```python
from build123d import *

# Parameters (mm, degrees)
SKETCH1_R             = 19.05
BOSS_EXTRUDE1_DEPTH   = 4.7625
SKETCH2_R             = 11.1125
BOSS_EXTRUDE2_DEPTH   = 1.5875
FILLET1_R             = 1.5875
CUT_EXTRUDE1_DEPTH    = 28.679008291
FILLET2_R             = 1.5875
F_4_40_TAPPED_HOLE1_D = 2.2606
CIRPATTERN1_COUNT     = 6
CHAMFER1_SIZE         = 0.762


with BuildPart() as part:
    # Sketch1 → Boss-Extrude1 (new body)
    with BuildSketch(Plane.XY):
        with Locations(Location((0, 0, 0), (0, 0, 180))):
            Circle(SKETCH1_R)
    extrude(amount=BOSS_EXTRUDE1_DEPTH)

    # Sketch2 → Boss-Extrude2 (add)
    with BuildSketch(Plane(origin=(0, 0, 0), x_dir=(-1, 0, 0), z_dir=(0, 0, -1))):
        with Locations(Location((0, 0, 0), (0, 0, 180))):
            Circle(SKETCH2_R)
    extrude(amount=BOSS_EXTRUDE2_DEPTH)

    # Fillet1
    fillet1_edges = [part.edges().sort_by_distance(p)[0] for p in [
        (-11.1125, 0, 0),
    ]]
    fillet(fillet1_edges, radius=FILLET1_R - 0.0001)  # a hair under: the kernel refuses the full size

    # Sketch3 → Cut-Extrude1 (cut, through all)
    with BuildSketch(Plane(origin=(0, 0, -1.5875), x_dir=(-1, 0, 0), z_dir=(0, 0, -1))):
        with BuildLine():
            Line((-4.7625, 4.200130206), (-4.7625, -4.200130206))
            ThreePointArc((-4.7625, -4.200130206), (0, -6.35), (4.7625, -4.200130206))
            Line((4.7625, -4.200130206), (4.7625, 4.200130206))
            ThreePointArc((4.7625, 4.200130206), (0, 6.35), (-4.7625, 4.200130206))
        make_face()
    extrude(amount=-CUT_EXTRUDE1_DEPTH, mode=Mode.SUBTRACT)

    # Fillet2
    fillet2_edges = [part.edges().sort_by_distance(p)[0] for p in [
        (4.7625, 4.200130206, 1.5875),
        (-4.7625, 4.200130206, 1.5875),
        (-4.7625, -4.200130206, 1.5875),
        (4.7625, -4.200130206, 1.5875),
    ]]
    fillet(fillet2_edges, radius=FILLET2_R)

    # #4-40 Tapped Hole1 (through all)
    with Locations(Plane.XY.offset(4.7625)):
        with Locations((0, 15.24)):
            f_4_40_tapped_hole1 = Hole(F_4_40_TAPPED_HOLE1_D / 2)

    # CirPattern1: #4-40 Tapped Hole1 ×6 about axis
    cirpattern1_axis = Axis((0, 0, 0), (0, 0, 1))
    for i in range(1, CIRPATTERN1_COUNT):
        add(f_4_40_tapped_hole1.rotate(cirpattern1_axis, i * 360 / CIRPATTERN1_COUNT), mode=Mode.SUBTRACT)

    # Chamfer1
    chamfer1_edges = [part.edges().sort_by_distance(p)[0] for p in [
        (-4.7625, 0, -1.5875),
        (0, -6.35, -1.5875),
        (4.7625, 0, -1.5875),
        (0, 6.35, -1.5875),
        (-4.6241826, -4.197852075, -1.5875),
        (4.6241826, -4.197852075, -1.5875),
        (-4.6241826, 4.197852075, -1.5875),
        (4.6241826, 4.197852075, -1.5875),
    ]]
    chamfer(chamfer1_edges, length=CHAMFER1_SIZE)


solid = part.part
```
Input: part model. Units: mm. Frame: model coordinates. A direction names the side the tool comes from. Round coordinates to 2 decimals unless told otherwise and drop trailing zeros. Write each loop counter-clockwise with the first axis right and the second up, starting at its lowest first coordinate (ties: lowest second). Pieces come first, ordered by that corner, then holes. Notation, with made-up numbers: (-21, -38.5) -> (-15, -38.5) arc R21 cw to (-15, -16.5) -> close; hole circle Ø3 at (82, -30.5). An arc over 180 degrees is marked (long way). Answer as CSV lines item,"result".
1. Contact query for flat-ended pins moving along their axis: P1, Ø4, axis at x = -14.5, y = -8.5, coming from the -Z side; P2, Ø1.4, axis at x = 13.2, y = -7.62, coming from the -Z side; P3, Ø8, axis at x = -7.5, y = -13.5, coming from the -Z side; P4, Ø3, axis at x = 3.5, z = 1, coming from the +Y side. Output: stop coordinate, or through.
Geometry says:
P1,"stops at z = 0"
P2,"passes through"
P3,"stops at z = -0.62"
P4,"stops at y = 18.94"
2. Reachability of faces 4 (the cylindrical face through (4.628, 4.189, 2.008)), 5 (the flat face through (5, -5, 4.762)) from +Z, -Z, +X, -X, +Y, -Y: full face, straight path, thin tool, end or side. Return the list, or none.
Geometry says:
face 4,"+Z, -Z"
face 5,"+Z, +X, -X, +Y, -Y"
3. Section B-B (y = 15.24). Return the cut outline in (x, z), plus the area to 3 significant figures.
Geometry says:
outline,"(-11.43, 0) -> (-1.13, 0) -> (-1.13, 4.76) -> (-11.43, 4.76) -> close; (1.13, 0) -> (11.43, 0) -> (11.43, 4.76) -> (1.13, 4.76) -> close"
area,"98.1 mm^2"
4. Mould query, pull axis Y, two halves, no side actions, for faces 1 (the cylindrical face through (4.13, 18.597, 2.348)), 2 (the flat face through (-12.4, 4, 0)), 3 (the cylindrical face through (0.06, -6.35, 1.93)). Classes: +Y half, -Y half, draft (parallel to the pull), parting line (faces both ways), or undercut.
Geometry says:
face 1,"parting line"
face 2,"draft"
face 3,"undercut"
5. Ray query, L1, parallel to Y at x = 0, z = 4.25; L2, parallel to X at y = -7, z = 2; L3, parallel to Y at x = -14, z = 3.25. Return the intervals inside material, ascending. Write a range as [from, to].
Geometry says:
L1,"y = [-19.05, -16.37], [-14.11, -6.35], [6.35, 14.11], [16.37, 19.05]"
L2,"x = [-17.72, -14.14], [-12.25, 12.25], [14.14, 17.72]"
L3,"y = [-12.92, -8.42], [-6.82, 6.82], [8.42, 12.92]"
6. Section A-A (x = 0). Give the number of separate pieces and of enclosed holes in the cut face, plus the area to 3 significant figures.
Geometry says:
separate pieces,"4"
enclosed holes,"0"
area,"115 mm^2"
